Autodesk Inventor part; units mm, degrees
ref_plane "bolt_XY" through (0, 0, 0) normal (1, 0, 0) x (0, 0, -1)
ref_plane "bolt_YZ" through (0, 0, 0) normal (0, 0, -1) x (0, 1, 0)
ref_plane "bolt_ZX" through (0, 0, 0) normal (0, 1, 0) x (1, 0, 0)
sketch "Sketch_1" plane through (0, 0, 0) normal (0, 0, 1) x (1, 0, 0)
  line L0 (8, 0) -> (-4, 0)
  line L1 (-4, 0) -> (-4, 3.5)
  line L2 (-4, 3.5) -> (0, 3.5)
  line L3 (0, 3.5) -> (0, 2)
  line L4 (0, 2) -> (7.5705, 2)
  line L5 (7.5705, 2) -> (8, 1.5705)
  line L6 (8, 1.5705) -> (8, 0)
  line L7 (8, 0) -> (-4, 0)
revolve "Revolution1" add sketch "Sketch_1" angle 360 about axis through (8, 0, 0) along (1, 0, 0)
thread "Thread1"
sketch "Sketch_4" plane through (0, 0, 0) normal (0, 0, 1) x (1, 0, 0)
  line L0 (-1.5981, 0) -> (-4, 0)
  line L1 (-4, 0) -> (-4, 1.5)
  line L2 (-4, 1.5) -> (-2, 1.5)
  line L3 (-2, 1.5) -> (-1.5981, 0)
  line L4 (-1.5981, 0) -> (-4, 0)
revolve "Revolution2" cut sketch "Sketch_4" angle 360 about axis through (-1.5981, 0, 0) along (1, 0, 0)
sketch "Sketch_3" plane through (-4, 0, 0) normal (1, 0, 0) x (0, 0, -1)
  line L0 (-1.5, 0.866) -> (-1.5, -0.866)
  line L1 (-1.5, -0.866) -> (0, -1.7321)
  line L2 (0, -1.7321) -> (1.5, -0.866)
  line L3 (1.5, -0.866) -> (1.5, 0.866)
  line L4 (1.5, 0.866) -> (0, 1.7321)
  line L5 (0, 1.7321) -> (-1.5, 0.866)
extrude "Extrusion1" cut sketch "Sketch_3" along normal blind 2
ref_plane "bolt_XY" through (0, 0, 0) normal (1, 0, 0) x (0, 0, -1)
ref_plane "bolt_YZ" through (0, 0, 0) normal (0, 0, -1) x (0, 1, 0)
ref_plane "bolt_ZX" through (0, 0, 0) normal (0, 1, 0) x (1, 0, 0)
ref_plane "nut_XY" through (8, 0, 0) normal (1, 0, 0) x (0, 0, -1)
ref_plane "nut_YZ" through (8, 0, 0) normal (0, 0, -1) x (0, 1, 0)
ref_plane "nut_ZX" through (8, 0, 0) normal (0, 1, 0) x (1, 0, 0)
properties part number "CBM4-8" material "MISUMI"
The listing builds one solid part. Answer for the finished solid, in the listing's coordinates (mm). A direction names the side the tool comes from. Give positions to 0.01 mm unless a question says otherwise; leave off trailing zeros. Loops run counter-clockwise (first coordinate to the right, second up) from the corner with the lowest first, then second, coordinate; pieces in that order, holes last. Notation, with made-up numbers: (85.5, 81) - (129.5, 81) arc R22 ccw to (129.5, 106) - close; hole circle Ø11 at (52.5, 40). An arc over 180 degrees is marked (long way). Answer as a JSON object with one key per item and string values.
1. Flat-ended cylindrical pins translate along their axes: pin 1 Ø3 at (x, z) = (5.5, 1) entering from +Y; pin 2 Ø2 at (x, z) = (0.5, -1) entering from +Y. Find the tip coordinate at first contact, or state that the pin passes through.
Determined:
{"pin 1": "y = 2", "pin 2": "y = 3.5"}
2. Find the intervals of material crossed by L1, parallel to X at y = 0.5, z = 2.75; L2, parallel to Z at x = 4, y = -1; L3, parallel to Y at x = -2.75, z = -1, in increasing order. Write a range as [from, to].
Determined:
{"L1": "[-4, 0]", "L2": "[-1.73, 1.73]", "L3": "[-3.35, -1.15], [1.15, 3.35]"}
3. For faces 1 (the flat face through (-3.014, -1.305, -0.74)), 2 (the cylindrical face through (-1.972, 3.233, -1.341)), 3 (the flat face through (0, 2, -2)), determine the directions among +Z, -Z, +X, -X, +Y, -Y from which every point of the face is accessible in a straight line to the end or side of a thin tool.
Determined:
{"face 1": "-X", "face 2": "+X, -X", "face 3": "+X"}
4. A cutting plane is placed at A-A (x = 3.25). Write down the section's boundary in (y, z), then the cut area to 3 significant figures.
Determined:
{"outline": "circle Ø4 at (0, 0)", "area": "12.6 mm²"}
5. For a pull along Y with two mould halves and no side action, classify faces 4 (the flat face through (8, 0, 0)), 5 (the cylindrical face through (4, 0, -2)), 6 (the flat face through (-3.014, -1.293, 0.76)) as pulls with the +Y half, pulls with the -Y half, needs draft (parallel to the pull), parting line crosses it, or undercut.
Determined:
{"face 4": "needs draft", "face 5": "parting line crosses it", "face 6": "undercut"}
6. A cutting plane is placed at B-B (y = 2.5). Write down the section's boundary in (x, z).
Determined:
{"outline": "(-4, -2.45) - (0, -2.45) - (0, 2.45) - (-4, 2.45) - close"}
